For this review, take the finished solid that the model builds, in its own axes (mm). A direction names the side the tool comes from. Give positions to 0.01 mm unless a question says otherwise; leave off trailing zeros. Loops run counter-clockwise (first coordinate to the right, second up) from the corner with the lowest first, then second, coordinate; pieces in that order, holes last. Notation, with made-up numbers: (-1.5, -23.75) - (19.5, -23.75) arc R32 ccw to (19.5, 5.25) - close; hole circle Ø8 at (67.25, 53.25). An arc over 180 degrees is marked (long way). Put each result on its own line as item: value.
from build123d import *

# Parameters (mm, degrees)
PAD003_DEPTH    = 5
SKETCH008_W     = 2
SKETCH008_H     = 5
POCKET004_DEPTH = 5
SKETCH009_R     = 2
POCKET005_DEPTH = 4


with BuildPart() as part:
    # Sketch007 → Pad003 (new body)
    with BuildSketch(Plane.XY):
        with BuildLine():
            ThreePointArc((5, 8.660254), (-10, 0), (5, -8.660254))
            Line((5, 8.660254), (5, -8.660254))
        make_face()
    extrude(amount=PAD003_DEPTH)

    # Sketch008 → Pocket004 (cut)
    with BuildSketch(Plane.XY.offset(5)):
        with Locations((-4, 4.5)):
            Rectangle(SKETCH008_W, SKETCH008_H)
        with Locations((3, 4.5)):
            Rectangle(SKETCH008_W, SKETCH008_H)
        with Locations((3, -4.5)):
            Rectangle(SKETCH008_W, SKETCH008_H)
        with Locations((-4, -4.5)):
            Rectangle(SKETCH008_W, SKETCH008_H)
    extrude(amount=-POCKET004_DEPTH, mode=Mode.SUBTRACT)

    # Sketch009 → Pocket005 (cut)
    with BuildSketch(Plane.XY.offset(5)):
        Circle(SKETCH009_R)
    extrude(amount=-POCKET005_DEPTH, mode=Mode.SUBTRACT)


solid = part.part
1) Take a section at D-D on y = 0. State the section outline as (x, z) points.
Geometry check:
outline: (-10, 0) - (5, 0) - (5, 5) - (2, 5) - (2, 1) - (-2, 1) - (-2, 5) - (-10, 5) - close
2) Take a section at B-B on z = 0.65. State the section outline as (x, y) points, and give its area (3 significant figures).
Geometry check:
outline: (5, -8.66) - (5, 8.66) arc R10 ccw (long way) to start; hole (-5, -7) - (-3, -7) - (-3, -2) - (-5, -2) - close; hole (-5, 2) - (-3, 2) - (-3, 7) - (-5, 7) - close; hole (2, -7) - (4, -7) - (4, -2) - (2, -2) - close; hole (2, 2) - (4, 2) - (4, 7) - (2, 7) - close
area: 213 mm²
3) Take a section at A-A on y = 5. State the section outline as (x, z) points.
Geometry check:
outline: (-8.66, 0) - (-5, 0) - (-5, 5) - (-8.66, 5) - close; (-3, 0) - (2, 0) - (2, 5) - (-3, 5) - close; (4, 0) - (5, 0) - (5, 5) - (4, 5) - close
4) Draft analysis for pull direction X (two halves, no side actions). For faces 4 (the face through (5, 0, 2)), 5 (the face through (-3, 0, 0)), 6 (the face through (3, -2, 3)), state which applies: pulls with the +X half, pulls with the -X half, needs draft (parallel to the pull), parting line crosses it, or undercut.
Geometry check:
face 4: pulls with the +X half
face 5: needs draft
face 6: undercut
5) Wall thickness on line 1 (X direction, y = 5, z = 4.5); line 2 (Y direction, x = 0, z = 2.9); line 3 (Y direction, x = 2.25, z = 2.85): over which ranges is each line inside the solid? List them lowest first.
Geometry check:
line 1: x = -8.66 to -5, -3 to 2, 4 to 5
line 2: y = -10 to -2, 2 to 10
line 3: y = -9.74 to -7, -2 to 2, 7 to 9.74
6) For faces 1 (the face through (-5, -5, 3)), 2 (the face through (-3, 0, 5)), 3 (the face through (0, 0, 1)), list the 3-axis set-ups (+Z, -Z, +X, -X, +Y, -Y) from which the entire face can be reached by the end or side of a thin tool; tool diameter is ignored.
Geometry check:
face 1: +Z, -Z
face 2: +Z, +X, -X, +Y, -Y
face 3: +Z
7) Insertion check: pin 1 Ø1.6 at (x, z) = (-4, 3) entering from +Y; pin 2 Ø0.6 at (x, z) = (3, 1.5) entering from -Y; pin 3 Ø2 at (x, z) = (-4.5, 2) entering from -Y. Each pin has a flat end and moves straight along its axis. Give the tip position at first contact, or say it passes through.
Geometry check:
pin 1: stops at y = 9.47
pin 2: stops at y = -9.63
pin 3: stops at y = -9.37
8) Take a section at C-C on x = -4. State the section outline as (y, z) points.
Geometry check:
outline: (-9.17, 0) - (-7, 0) - (-7, 5) - (-9.17, 5) - close; (-2, 0) - (2, 0) - (2, 5) - (-2, 5) - close; (7, 0) - (9.17, 0) - (9.17, 5) - (7, 5) - close
